Source: three-view drawing plus pictorial views. Frame: mm from the lowest corner of the part. A direction names the side the tool comes from. Give positions to 0.01 mm unless a question says otherwise; leave off trailing zeros. Loops run counter-clockwise (first coordinate to the right, second up) from the corner with the lowest first, then second, coordinate; pieces in that order, holes last. Notation, with made-up numbers: M 33.5,29 L 37.5,29 A22 cw 37.5,50 Z; hole C 19.25,-8.75 d7. An arc over 180 degrees is marked long. One line per item, written item: value. Start each with the question number.
(1) Access query for the marked faces 4 and 5. Directions: +Z, -Z, +X, -X, +Y, -Y. A direction counts if a zero-diameter tool reaches every point of the face in a straight line with its end or side. Return the directions, or none.
(2) Pin query (flat end, axial travel): P1, Ø1.3, axis at y = 3.5, z = 3, coming from the -X side; P2, Ø1.5, axis at x = 13.5, z = 3, coming from the -Y side. Return the tip coordinate at first contact, or that it passes through.
(3) Section C-C on y = 4. Output: boundary loops of the cut face in (x, z).
(4) Pull-direction query (Y, two-part tool) for the marked faces 1, 2 and 3; classes: released by +Y, released by -Y, zero draft, split by the parting line, or undercut.
(5) Section D-D on x = 1.75. Output: boundary loops of the cut face in (y, z), plus the area to 3 significant figures.
(6) Section A-A on x = 12. Output: boundary loops of the cut face in (y, z).
(7) Section B-B on z = 3. Output: boundary loops of the cut face in (x, y).
(8) Ray query, line 1 along Z through (x, y) = (2.75, 4); line 2 along X through (y, z) = (0.5, 0.3); line 3 along Y through (x, z) = (13.5, 5). Return the intervals inside material, ascending. Write a range as from..to.
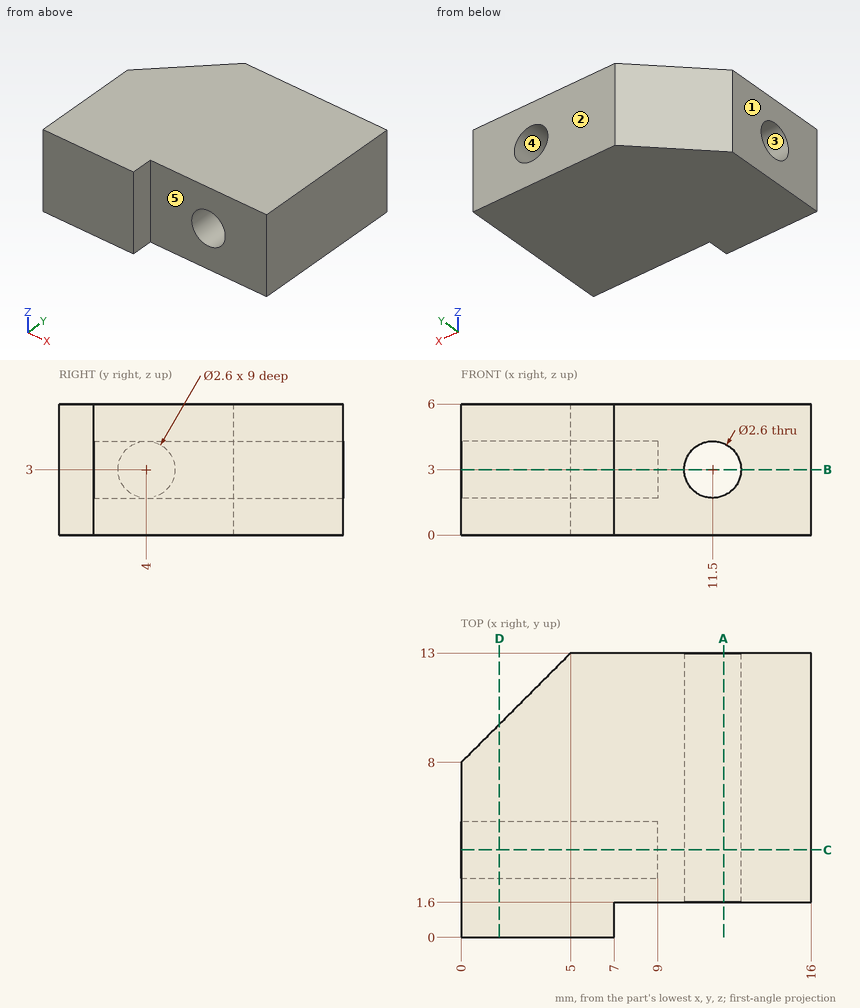
Output values:
1. face 4: +Y, -Y
1. face 5: +Z, -Z, +X, -Y
2. P1: stops at x = 9
2. P2: stops at y = 1.6
3. outline: M 0,0 L 16,0 L 16,6 L 0,6 L 0,4.3 L 9,4.3 L 9,1.7 L 0,1.7 Z; hole C 11.5,3 d2.6
4. face 1: zero draft
4. face 2: released by +Y
4. face 3: undercut
5. outline: M 0,0 L 9.75,0 L 9.75,6 L 0,6 Z; hole C 4,3 d2.6
5. area: 53.2 mm²
6. outline: M 1.6,0 L 13,0 L 13,1.8 L 1.6,1.8 Z; M 1.6,4.2 L 13,4.2 L 13,6 L 1.6,6 Z
7. outline: M 0,0 L 7,0 L 7,1.6 L 10.2,1.6 L 10.2,13 L 5,13 L 0,8 L 0,5.3 L 9,5.3 L 9,2.7 L 0,2.7 Z; M 12.8,1.6 L 16,1.6 L 16,13 L 12.8,13 Z
8. line 1: z = 0..1.7, 4.3..6
8. line 2: x = 0..7
8. line 3: y = 1.6..13
